from build123d import *

# Parameters (mm, degrees)
F1_DEPTH  = 105
F2_R      = 2.75
F2_R_2    = 3.342639
F3_DEPTH  = 20.001
F5_DEPTH  = 25.001
F7_DEPTH  = 5
F9_DEPTH  = 7
F10_R     = 4
F11_DEPTH = 2.2
F12_R     = 5
F13_DEPTH = 7
F15_DEPTH = 3


with BuildPart() as f1:
    # F0 (on Front) → F1 (new body, symmetric)
    with BuildSketch(Plane.XZ):
        Polygon((-12.5, -6.5), (-12.5, -10), (12.5, -10), (12.5, 10), (-5.7, 10), (-5.7, -6.5), align=None)
    extrude(amount=F1_DEPTH, both=True)

    # F2 (on face) → F3 (cut, through all)
    with BuildSketch(Plane.XY.offset(10)):
        with Locations((0, 80)):
            Circle(F2_R)
        with Locations((0, -80)):
            Circle(F2_R_2)
    extrude(amount=-F3_DEPTH, mode=Mode.SUBTRACT)

    # F4 (on face) → F5 (cut, through all)
    with BuildSketch(Plane.YZ.offset(12.5)):
        with BuildLine():
            ThreePointArc((-65, 4.25), (-66.944544, 3.444544), (-67.75, 1.5))
            Line((-67.75, 1.5), (-67.75, -0.5))
            ThreePointArc((-67.75, -0.5), (-66.944544, -2.444544), (-65, -3.25))
            ThreePointArc((-65, -3.25), (-63.055456, -2.444544), (-62.25, -0.5))
            Line((-62.25, -0.5), (-62.25, 1.5))
            ThreePointArc((-62.25, 1.5), (-63.055456, 3.444544), (-65, 4.25))
        make_face()
        with BuildLine():
            ThreePointArc((65, 4.25), (63.055456, 3.444544), (62.25, 1.5))
            Line((62.25, 1.5), (62.25, -0.5))
            ThreePointArc((62.25, -0.5), (63.055456, -2.444544), (65, -3.25))
            ThreePointArc((65, -3.25), (66.944544, -2.444544), (67.75, -0.5))
            Line((67.75, -0.5), (67.75, 1.5))
            ThreePointArc((67.75, 1.5), (66.944544, 3.444544), (65, 4.25))
        make_face()
    extrude(amount=-F5_DEPTH, mode=Mode.SUBTRACT)

    # F6 (on face) → F7 (cut)
    with BuildSketch(Plane.YZ.offset(12.5)):
        with BuildLine():
            Line((-64.860655, -6), (-64.834395, -6))
            ThreePointArc((-64.834395, -6), (-60.902267, -4.345564), (-59.335758, -0.377587))
            Line((-59.335758, -0.377587), (-59.380282, 1.622413))
            ThreePointArc((-59.380282, 1.622413), (-61.033355, 5.432129), (-64.87892, 7))
            Line((-64.87892, 7), (-64.905179, 7))
            ThreePointArc((-64.905179, 7), (-68.837308, 5.345564), (-70.403817, 1.377587))
            Line((-70.403817, 1.377587), (-70.359292, -0.622413))
            ThreePointArc((-70.359292, -0.622413), (-68.706219, -4.432129), (-64.860655, -6))
        make_face()
        with BuildLine():
            Line((59.380282, 1.622413), (59.335758, -0.377587))
            ThreePointArc((59.335758, -0.377587), (60.902267, -4.345564), (64.834395, -6))
            Line((64.834395, -6), (64.860655, -6))
            ThreePointArc((64.860655, -6), (68.706219, -4.432129), (70.359292, -0.622413))
            Line((70.359292, -0.622413), (70.403817, 1.377587))
            ThreePointArc((70.403817, 1.377587), (68.837308, 5.345564), (64.905179, 7))
            Line((64.905179, 7), (64.87892, 7))
            ThreePointArc((64.87892, 7), (61.033355, 5.432129), (59.380282, 1.622413))
        make_face()
    extrude(amount=-F7_DEPTH, mode=Mode.SUBTRACT)

    # F8 (on face) → F9 (cut)
    with BuildSketch(Plane(origin=(-5.7, 0, 0), x_dir=(0, -1, 0), z_dir=(-1, 0, 0))):
        with BuildLine():
            ThreePointArc((60, -1.5), (61.464466, -5.035534), (65, -6.5))
            ThreePointArc((65, -6.5), (68.535534, -5.035534), (70, -1.5))
            Line((70, -1.5), (70, 2.267072))
            ThreePointArc((70, 2.267072), (67.714856, 6.465829), (62.948177, 6.826679))
            ThreePointArc((62.948177, 6.826679), (60.801243, 4.981928), (60, 2.267072))
            Line((60, 2.267072), (60, -1.5))
        make_face()
        with BuildLine():
            ThreePointArc((67.75, -0.5), (65, -3.25), (62.25, -0.5))
            Line((62.25, -0.5), (62.25, 1.5))
            ThreePointArc((62.25, 1.5), (65, 4.25), (67.75, 1.5))
            Line((67.75, 1.5), (67.75, -0.5))
        make_face(mode=Mode.SUBTRACT)
        with BuildLine():
            ThreePointArc((-62.948177, 6.826679), (-67.714856, 6.465829), (-70, 2.267072))
            Line((-70, 2.267072), (-70, -1.5))
            ThreePointArc((-70, -1.5), (-68.535534, -5.035534), (-65, -6.5))
            ThreePointArc((-65, -6.5), (-61.464466, -5.035534), (-60, -1.5))
            Line((-60, -1.5), (-60, 2.267072))
            ThreePointArc((-60, 2.267072), (-60.801243, 4.981928), (-62.948177, 6.826679))
        make_face()
        with BuildLine():
            ThreePointArc((-62.25, -0.5), (-65, -3.25), (-67.75, -0.5))
            Line((-67.75, -0.5), (-67.75, 1.5))
            ThreePointArc((-67.75, 1.5), (-65, 4.25), (-62.25, 1.5))
            Line((-62.25, 1.5), (-62.25, -0.5))
        make_face(mode=Mode.SUBTRACT)
    extrude(amount=-F9_DEPTH, mode=Mode.SUBTRACT)

    # F10 (on face) → F11 (cut)
    with BuildSketch(Plane.XY.offset(10)):
        with Locations((0, -80)):
            Circle(F10_R)
        with Locations((0, 80)):
            Circle(F10_R)
    extrude(amount=-F11_DEPTH, mode=Mode.SUBTRACT)

    # F12 (on face) → F13 (cut)
    with BuildSketch(Plane(origin=(0, 0, -10), x_dir=(1, 0, 0), z_dir=(0, 0, -1))):
        with Locations((0, 80)):
            Circle(F12_R)
        with Locations((0, -80)):
            Circle(F12_R)
    extrude(amount=-F13_DEPTH, mode=Mode.SUBTRACT)

    # F14 (on face) → F15 (cut)
    with BuildSketch(Plane.YZ.offset(12.5)):
        with BuildLine():
            Line((20, 8), (-20, 8))
            ThreePointArc((-20, 8), (-24.242641, 6.242641), (-26, 2))
            ThreePointArc((-26, 2), (-24.242641, -2.242641), (-20, -4))
            Line((-20, -4), (20, -4))
            ThreePointArc((20, -4), (24.242641, -2.242641), (26, 2))
            ThreePointArc((26, 2), (24.242641, 6.242641), (20, 8))
        make_face()
    extrude(amount=-F15_DEPTH, mode=Mode.SUBTRACT)


solid = f1.part
Work out the finished part from the listing and answer in its coordinate system (mm). A direction names the side the tool comes from. Round coordinates to 2 decimals unless told otherwise and drop trailing zeros. Write each loop counter-clockwise with the first axis right and the second up, starting at its lowest first coordinate (ties: lowest second). Pieces come first, ordered by that corner, then holes. Notation, with made-up numbers: (55, 57) - (108, 57) arc R27 ccw to (108, 82) - close; hole circle Ø2 at (75.5, 18). An arc over 180 degrees is marked (long way). Answer in a Markdown table with one row per item. Add a question column.
1. Given pin 1 (5 mm diameter, centred on x = -1.5, y = 81, fed in from -Z); pin 2 (2 mm diameter, centred on x = -8.5, y = -38, fed in from +Z), each flat-ended and moving along its own axis, determine where each tip first touches the part or whether it passes through.
2. A cutting plane is placed at A-A, the plane y = 80. Determine the outline of the cut face in (x, z), and give its area (3 significant figures).
3. Find the intervals of material crossed by line 1 along Y through (x, z) = (0, -8.25); line 2 along Y through (x, z) = (4.75, -0.75); line 3 along Y through (x, z) = (0, 1), in increasing order. Write a range as from..to.
4. A cutting plane is placed at C-C, the plane y = -80. Determine the outline of the cut face in (x, z).
5. A cutting plane is placed at B-B, the plane y = 7. Determine the outline of the cut face in (x, z).
6. For faces 1 (the cylindrical face through (-1.08, -75.12, -6.55)), 2 (the flat face through (-2, 70, 0)), 3 (the flat face through (-9, -1, -6.5)), 4 (the flat face through (9.5, 0, 2)), 5 (the flat face through (12.5, -1, -5)), determine the directions among +Z, -Z, +X, -X, +Y, -Y from which every point of the face is accessible in a straight line to the end or side of a thin tool.
7. A cutting plane is placed at D-D, the plane x = -8.25. Determine the outline of the cut face in (y, z), and give its area (3 significant figures).
8. The mould has two halves that part along Z. Classify faces 6 (the cylindrical face through (-1.08, 84.88, -6.55)), 7 (the flat face through (4, -1, 10)), 8 (the cylindrical face through (10.035, 68.663, -4.474)): +Z half, -Z half, draft (parallel to the pull), parting line (faces both ways), or undercut.
Worked out:
| question | item | result |
|---|---|---|
| 1 | pin 1 | z = -3 |
| 1 | pin 2 | z = -6.5 |
| 2 | outline | (-12.5, -10) - (-5, -10) - (-5, -3) - (-2.75, -3) - (-2.75, 7.8) - (-4, 7.8) - (-4, 10) - (-5.7, 10) - (-5.7, -6.5) - (-12.5, -6.5) - close; (2.75, -3) - (5, -3) - (5, -10) - (12.5, -10) - (12.5, 10) - (4, 10) - (4, 7.8) - (2.75, 7.8) - close |
| 2 | area | 241 mm^2 |
| 3 | line 1 | -105..-85, -75..75, 85..105 |
| 3 | line 2 | -105..-67.74, -62.26..62.26, 67.74..105 |
| 3 | line 3 | -105..-83.34, -76.66..-70, -60..60, 70..77.25, 82.75..105 |
| 4 | outline | (-12.5, -10) - (-5, -10) - (-5, -3) - (-3.34, -3) - (-3.34, 7.8) - (-4, 7.8) - (-4, 10) - (-5.7, 10) - (-5.7, -6.5) - (-12.5, -6.5) - close; (3.34, -3) - (5, -3) - (5, -10) - (12.5, -10) - (12.5, 10) - (4, 10) - (4, 7.8) - (3.34, 7.8) - close |
| 5 | outline | (-12.5, -10) - (12.5, -10) - (12.5, -4) - (9.5, -4) - (9.5, 8) - (12.5, 8) - (12.5, 10) - (-5.7, 10) - (-5.7, -6.5) - (-12.5, -6.5) - close |
| 6 | face 1 | -Z |
| 6 | face 2 | -X |
| 6 | face 3 | +Z, -X, +Y, -Y |
| 6 | face 4 | +X |
| 6 | face 5 | +Z, -Z, +X, +Y, -Y |
| 7 | outline | (-105, -10) - (105, -10) - (105, -6.5) - (-105, -6.5) - close |
| 7 | area | 735 mm^2 |
| 8 | face 6 | draft |
| 8 | face 7 | +Z half |
| 8 | face 8 | undercut |
